Autodesk Inventor part; units mm, degrees
ref_plane "YZ Plane" through (0, 0, 0) normal (1, 0, 0) x (0, 1, 0)
ref_plane "XZ Plane" through (0, 0, 0) normal (0, 1, 0) x (-1, 0, 0)
ref_plane "XY Plane" through (0, 0, 0) normal (0, 0, 1) x (1, 0, 0)
sketch "Sketch1" plane through (0, 0, 0) normal (0, 1, 0) x (-1, 0, 0)
  line L0 (0, 0) -> (0, -32)
  line L1 (0, -32) -> (52, -32)
  line L2 (52, -32) -> (52, -30)
  line L3 (52, -30) -> (2, -30)
  line L4 (2, -30) -> (2, 0)
  line L5 (2, 0) -> (0, 0)
  dimension "d0" = 2
  dimension "d1" = 2
  dimension "d2" = 50
  dimension "d3" = 30
extrude "base" add sketch "Sketch1" along normal blind 20
sketch "Sketch2" plane through (-52, 0, -30) normal (0, 0, 1) x (1, 0, 0)
  line L0 (0, 0) -> (50, 0) construction
  line L1 (50, 0) -> (50, 20) construction
  line L2 (0, 20) -> (50, 20) construction
  line L3 (0, 0) -> (0, 20) construction
  line L4 (0, 0) -> (50, 0) construction
  line L5 (52, 20) -> (0, 20) construction
  circle A0 centre (15, 10) radius 2.5
  line L6 (0, 0) -> (0, 20)
  line L7 (0, 10) -> (52, 10)
  line L8 (52, 0) -> (52, 20)
  dimension "d6" = 5
  dimension "d9" = 15
extrude "shaftHole" cut sketch "Sketch2" against normal blind 30
sketch "Sketch4" plane through (0, 0, 0) normal (1, 0, 0) x (0, 0, -1)
  line L0 (32, 0) -> (32, 20) construction
  line L1 (0, 0) -> (0, 20) construction
  line L2 (30, 0) -> (30, 20) construction
  line L3 (0, 10) -> (30, 10) construction
  line L4 (9, 5) -> (9, 15) construction
  line L5 (19, 15) -> (19, 5) construction
  point P0 (9, 10)
  point P1 (19, 10)
  dimension "d22" = 30
  dimension "d29" = 10
  dimension "d30" = 9
  dimension "d31" = 10
  dimension "d32" = 10
hole "Hole1" at (0, 5, -9) at (0, 15, -9) at (0, 15, -19) at (0, 5, -19) direction (-1, 0, 0) diameter 5 end through all
equation "\"d1\" = d0"
equation "\"d31\" = d29"
properties part number "motorBracket" material "Steel"
The model under review builds one solid part; all positions refer to its coordinate system, in mm. A direction names the side the tool comes from. Give positions to 0.01 mm unless a question says otherwise; leave off trailing zeros. Order: outer loops, then holes, each group sorted by start corner. A loop starts at its lowest first (then second) coordinate and runs counter-clockwise, first axis right, second up. Notation, with made-up numbers: M -2,32.25 L 24,32.25 A23 cw 24,63.25 Z; hole C 19.5,48 d11. An arc over 180 degrees is marked long. Use one line per item in the form item = value. Start each with the question number.
Item 1: We need section A-A on y = 5. Give the boundary of the cut face in (x, z), plus the area to 3 significant figures.
Item 2: To check wall thickness, follow line 1 along Y through (x, z) = (-1.1, -9); line 2 along Z through (x, y) = (-0.7, 5); line 3 along Z through (x, y) = (-28, 14.25). State the ranges of each line that lie inside material, in increasing order. Write a range as from..to.
Item 3: We need section B-B on z = -17.5. Give the boundary of the cut face in (x, y), plus the area to 3 significant figures.
Item 4: For faces 1 (the flat face through (-2, 10, -15)), 2 (the cylindrical face through (-34.69, 9.04, -30.99)), list the 3-axis set-ups (+Z, -Z, +X, -X, +Y, -Y) from which the entire face can be reached by the end or side of a thin tool; tool diameter is ignored.
Item 5: We need section D-D on y = 10. Give the boundary of the cut face in (x, z).
Item 6: The part is to be moulded in two halves that separate along Z. For faces 3 (the cylindrical face through (-1, 4.9, -16.5)), 4 (the flat face through (-52, 10, -31)), 5 (the flat face through (-26, 10, -32)), 6 (the flat face through (-27, 10, -30)), say which applies: pulls with the +Z half, pulls with the -Z half, needs draft (parallel to the pull), parting line crosses it, or undercut.
Item 7: We need section C-C on x = -37. Give the boundary of the cut face in (y, z).
Item 8: Insertion check: pin 1 Ø5 at (y, z) = (16, -12.5) entering from -X; pin 2 Ø8 at (x, y) = (-37, 10) entering from -Z; pin 3 Ø4.5 at (y, z) = (5, -9) entering from -X. Each pin has a flat end and moves straight along its axis. Give the tip position at first contact, or say it passes through.
Completed:
q1.outline = M -52,-32 L 0,-32 L 0,-21.5 L -2,-21.5 L -2,-30 L -52,-30 Z; M -2,-16.5 L 0,-16.5 L 0,-11.5 L -2,-11.5 Z; M -2,-6.5 L 0,-6.5 L 0,0 L -2,0 Z
q1.area = 144 mm²
q2.line_1 = 0..2.5, 7.5..12.5, 17.5..20
q2.line_2 = -32..-21.5, -16.5..-11.5, -6.5..0
q2.line_3 = -32..-30
q3.outline = M -2,0 L 0,0 L 0,3 L -2,3 Z; M -2,7 L 0,7 L 0,13 L -2,13 Z; M -2,17 L 0,17 L 0,20 L -2,20 Z
q3.area = 24.0 mm²
q4.face_1 = +Z, -X, +Y, -Y
q4.face_2 = +Z, -Z
q5.outline = M -52,-32 L -39.5,-32 L -39.5,-30 L -52,-30 Z; M -34.5,-32 L 0,-32 L 0,0 L -2,0 L -2,-30 L -34.5,-30 Z
q6.face_3 = undercut
q6.face_4 = needs draft
q6.face_5 = pulls with the -Z half
q6.face_6 = pulls with the +Z half
q7.outline = M 0,-32 L 7.5,-32 L 7.5,-30 L 0,-30 Z; M 12.5,-32 L 20,-32 L 20,-30 L 12.5,-30 Z
q8.pin_1 = -2
q8.pin_2 = -32
q8.pin_3 = through
